Autodesk Inventor part; units mm, degrees
ref_plane "YZ Plane" through (0, 0, 0) normal (1, 0, 0) x (0, 1, 0)
ref_plane "XZ Plane" through (0, 0, 0) normal (0, 1, 0) x (-1, 0, 0)
ref_plane "XY Plane" through (0, 0, 0) normal (0, 0, 1) x (1, 0, 0)
sketch "草图1" plane through (0, 0, 0) normal (0, 0, 1) x (1, 0, 0)
  line L0 (-5, 0) -> (5, 0) construction
  line L1 (-5, -6.3307) -> (5, -6.3307)
  line L2 (5, 5.4693) -> (-5, 5.4693)
  arc A0 (-5, 5.4693) -> (-5, -6.3307) centre (-1.0059, -0.4307) ccw
  line L3 (0, 0) -> (0, 3.0217)
  arc A1 (5, -6.3307) -> (5, 5.4693) centre (1.0059, -0.4307) ccw
  line L4 (5, 5.4693) -> (5, -6.3307)
  line L5 (-5, 5.4693) -> (-5, -6.3307)
  point P0 (-10.9, 0)
  point P1 (10.9, 0)
  point P2 (10.9, 0)
  dimension "d0" = 11.8
  dimension "d6" = 10
extrude "拉伸1" add sketch "草图1" along normal blind 29
sketch "草图2" plane through (0, 0, 29) normal (0, 0, 1) x (1, 0, 0)
  line L0 (6, -5.4307) -> (-6, -5.4307)
  line L1 (-6, -5.4307) -> (-6, 4.5693)
  line L2 (-6, 4.5693) -> (6, 4.5693)
  line L3 (6, 4.5693) -> (6, -5.4307)
  line L4 (6, -5.4307) -> (-6, 4.5693) construction
  line L5 (-6, -5.4307) -> (6, 4.5693) construction
  line L6 (5, 5.4693) -> (-5, 5.4693)
  line L7 (0, 5.4693) -> (0, -6.3307)
  line L8 (-5, -6.3307) -> (5, -6.3307)
  point P0 (0, -0.4307)
  dimension "d4" = 10
  dimension "d5" = 12
extrude "拉伸2" add sketch "草图2" along normal blind 18
sketch "草图3" plane through (0, 0, 0) normal (0, 0, -1) x (-1, 0, 0)
  line L0 (5, -6.3307) -> (-5, -6.3307)
  arc A0 (5, -6.3307) -> (5, 5.4693) centre (1.0059, -0.4307) ccw
  line L1 (-5, 5.4693) -> (5, 5.4693)
  arc A1 (-5, 5.4693) -> (-5, -6.3307) centre (-1.0059, -0.4307) ccw
  arc A2 (5.2957, -7.3307) -> (5.2957, 6.4693) centre (1.0059, -0.4307) ccw
  line L2 (5.2957, -7.3307) -> (-5.2957, -7.3307)
  arc A3 (-5.2957, 6.4693) -> (-5.2957, -7.3307) centre (-1.0059, -0.4307) ccw
  line L3 (-5.2957, 6.4693) -> (5.2957, 6.4693)
  line L4 (-9.1307, -0.4307) -> (9.1307, -0.4307)
  line L5 (9.1307, -0.4307) -> (9.1307, -12.0307)
  line L6 (9.1307, -12.0307) -> (-9.1307, -12.0307)
  line L7 (-9.1307, -12.0307) -> (-9.1307, -0.4307)
  point P0 (0, 0)
  dimension "d9" = 1
  dimension "d10" = 18.5
extrude "拉伸3" add sketch "草图3" along normal blind 1
sketch "草图4" plane through (0, 0, -1) normal (0, 0, -1) x (-1, 0, 0)
  circle A0 centre (0, 0) radius 5.5587
extrude "拉伸4" add sketch "草图4" along normal blind 2
sketch "草图5" plane through (-6, -5.4307, 29) normal (0, 1, 0) x (1, 0, 0)
  circle A0 centre (6, -14) radius 1.5
  line L0 (12, -18) -> (0, -18)
  point P0 (6, 29)
  dimension "d15" = 4
  dimension "d16" = 3
extrude "拉伸5" add sketch "草图5" against normal blind 8
sketch "草图7" plane through (0, -13.4307, 43) normal (0, -1, 0) x (1, 0, 0)
  circle A0 centre (0, 0) radius 1.5
  line L0 (-1.118, 1) -> (1.118, 1)
  point P0 (0, -43)
  point P1 (0, 1.5)
  dimension "d19" = 0.5
extrude "拉伸6" cut sketch "草图7" against normal up to surface (8 mm away) contours L0 A0 picked at (-0.0599, 1.1631)
fillet "圆角1" radius 4 4 edges at (-5, 5.4693, 14.5) (5, 5.4693, 14.5) (-5, -6.3307, 14.5) (5, -6.3307, 14.5)
fillet "圆角2" radius 3 2 edges at (-9.1307, -12.0307, -0.5) (9.1307, -12.0307, -0.5)
sketch "草图8" plane through (-6, -5.4307, 29) normal (0, -1, 0) x (1, 0, 0)
  circle A0 centre (10.0294, 16.2) radius 0.7
  circle A1 centre (1.5294, 16.2) radius 0.7
  line L0 (0, 18) -> (12, 18)
  point P0 (6, -29)
  dimension "d24" = 1.4
  dimension "d25" = 1.4
  dimension "d26" = 8.5
  dimension "d27" = 1.8
extrude "拉伸7" cut sketch "草图8" against normal blind 11.75
sketch "草图9" plane through (-6, 4.5693, 29) normal (0, 1, 0) x (1, 0, 0)
  line L0 (6, -14) -> (6, -2)
  circle A0 centre (6, -2) radius 1.5
  arc A1 (8.5, -14) -> (3.5, -14) centre (6, -14) ccw
  point P0 (6, 29)
  dimension "d30" = 12
  dimension "d31" = 3
extrude "拉伸8" cut sketch "草图9" against normal blind 23
sketch "草图10" plane through (0, 0, 29) normal (0, 0, 1) x (1, 0, 0)
  line L0 (-6, 4.5693) -> (6, 4.5693)
  line L1 (0, 4.5693) -> (0, -5.4307)
  line L2 (6, -5.4307) -> (-6, -5.4307)
  line L3 (8.5655, -4.9307) -> (-8.5655, -4.9307)
  line L4 (-8.5655, -4.9307) -> (-8.5655, 4.0693)
  line L5 (-8.5655, 4.0693) -> (8.5655, 4.0693)
  line L6 (8.5655, 4.0693) -> (8.5655, -4.9307)
  line L7 (8.5655, -4.9307) -> (-8.5655, 4.0693) construction
  line L8 (-8.5655, -4.9307) -> (8.5655, 4.0693) construction
  point P0 (0, 0)
  point P1 (0, -0.4307)
  dimension "d34" = 0.5
extrude "拉伸9" cut sketch "草图10" along normal blind 39.5
sketch "草图11" plane through (0, 0, 29) normal (0, 0, 1) x (1, 0, 0)
  circle A0 centre (0, -0.4307) radius 2.5
  arc A1 (-6.6623, 3.9014) -> (-6.6623, -4.7629) centre (-1.0059, -0.4307) ccw
  line L0 (-8.1307, -0.4307) -> (8.1307, -0.4307)
  arc A2 (6.6623, -4.7629) -> (6.6623, 3.9014) centre (1.0059, -0.4307) ccw
  dimension "d37" = 5
extrude "拉伸10" add sketch "草图11" along normal blind 6
sketch "草图12" plane through (0, 0, 29) normal (0, 0, 1) x (1, 0, 0)
  circle A0 centre (0, -0.4307) radius 5.831
  circle A1 centre (5, 2.5693) radius 1
  circle A2 centre (0, -0.4307) radius 5.5587
  line L0 (0, -0.4307) -> (0, 11.5704)
  line L1 (0, -0.4307) -> (0, 11.9593)
  circle A3 centre (-5, 2.5693) radius 1
  line L2 (0, -0.4307) -> (-7.5185, -0.4307)
  circle A4 centre (-5, -3.4307) radius 1
  arc A5 (-6.6623, 3.9014) -> (-6.6623, -4.7629) centre (-1.0059, -0.4307) ccw
  line L3 (-8.1307, -0.4307) -> (8.1307, -0.4307)
  arc A6 (6.6623, -4.7629) -> (6.6623, 3.9014) centre (1.0059, -0.4307) ccw
  dimension "d40" = 2
  dimension "d41" = 5
  dimension "d42" = 3
extrude "拉伸11" cut sketch "草图12" against normal blind 6 contours A1 A2 A0 | A0 A1 | A4 A0 | A0 A4 A2 | A1 A2 | A2 A4
properties part number "电机"
Could you check a few things on this model? Use its own coordinates, in mm. A direction names the side the tool comes from. Round coordinates to 2 decimals unless told otherwise and drop trailing zeros. Loops run counter-clockwise (first coordinate to the right, second up) from the corner with the lowest first, then second, coordinate; pieces in that order, holes last. Notation, with made-up numbers: M -9,87.5 L 17,87.5 A24 ccw 17,100.5 Z; hole C 87,71.25 d9. An arc over 180 degrees is marked long. Write item = value, one per line.
1. I want a section at B-B, the plane z = 45.2. Write out the boundary of the cut face in (x, y).
Results below:
outline = M -6,-5.43 L -5.17,-5.43 L -5.17,-4.93 L -6,-4.93 Z; M -6,4.07 L -5.17,4.07 L -5.17,4.57 L -6,4.57 Z; M -3.77,-5.43 L 3.33,-5.43 L 3.33,-4.93 L -3.77,-4.93 Z; M -3.77,4.07 L 3.33,4.07 L 3.33,4.57 L -3.77,4.57 Z; M 4.73,-5.43 L 6,-5.43 L 6,-4.93 L 4.73,-4.93 Z; M 4.73,4.07 L 6,4.07 L 6,4.57 L 4.73,4.57 Z
2. I need wall thicknesses on probe 1 along X at (y, z) = (-5.2, 45.2); probe 2 along Y at (x, z) = (-4.25, 32.5); probe 3 along Z at (x, y) = (0, 4.25). Which ranges of each line are inside material? Lowest first, please.
Results below:
probe_1 = -6 to -5.17, -3.77 to 3.33, 4.73 to 6
probe_2 = -5.43 to -4.93, 4.07 to 4.57
probe_3 = -3 to 29.5, 32.5 to 47
3. Thinking about a two-plate mould opening in X: for faces 1 (the face through (-8.13, -0.5, 14.3)), 2 (the face through (-4.562, -5.184, 45.894)), 3 (the face through (4.4, 3.4, -2)), which applies, +X half, -X half, draft (parallel to the pull), parting line (faces both ways), or undercut?
Results below:
face_1 = -X half
face_2 = undercut
face_3 = parting line
4. I want a section at C-C, the plane z = 18.5. Write out the boundary of the cut face in (x, y), and give its area (3 significant figures).
Results below:
outline = M -6.66,-4.76 A4 ccw -3.49,-6.33 L 3.49,-6.33 A4 ccw 6.66,-4.76 A7.12 ccw 6.66,3.9 A4 ccw 3.49,5.47 L -3.49,5.47 A4 ccw -6.66,3.9 A7.12 ccw Z
area = 169 mm²
5. I want a section at A-A, the plane z = 31. Write out the boundary of the cut face in (x, y).
Results below:
outline = M -6,-5.43 L -1.5,-5.43 L -1.5,-4.93 L -6,-4.93 Z; M -6,4.07 L -1.5,4.07 L -1.5,4.57 L -6,4.57 Z; C 0,-0.43 d5; M 1.5,-5.43 L 6,-5.43 L 6,-4.93 L 1.5,-4.93 Z; M 1.5,4.07 L 6,4.07 L 6,4.57 L 1.5,4.57 Z
6. Which directions (+Z, -Z, +X, -X, +Y, -Y) give clear straight access to the entire face, cutting with the end or side of a thin tool? Please do faces 4 (the face through (-5.23, 5.07, 14.7)), 5 (the face through (-5.28, -5.906, 14.703)), 6 (the face through (0, -4.931, 38)).
Results below:
face_4 = +Z, -X, +Y
face_5 = +Z, -X, -Y
face_6 = +Z, +X, -X
7. I want a section at D-D, the plane y = -11. Write out the boundary of the cut face in (x, z), and give its area (3 significant figures).
Results below:
outline = M -8.39,-1 L 8.39,-1 L 8.39,0 L -8.39,0 Z; M -1.12,44 A1.5 ccw long 1.12,44 Z
area = 23.1 mm²
8. Will these pins go through, and if not, where does the flat tip stop? P1, Ø1.6, axis at x = -5, y = -3.43, coming from the +Z side; P2, Ø1, axis at y = 2, z = 19, coming from the -X side; P3, Ø2, axis at x = 4.03, z = 45.2, coming from the -Y side.
Results below:
P1 = 23
P2 = -7.86
P3 = -5.43
